Read the model definition and answer for the solid it produces. Units are mm, in the model's axes. Coordinates: 2 decimals unless noted, no trailing zeros. Write each loop counter-clockwise with the first axis right and the second up, starting at its lowest first coordinate (ties: lowest second). Pieces come first, ordered by that corner, then holes. Notation, with made-up numbers: (-24, 35.25) -> (11, 35.25) arc R33 ccw to (11, 69.25) -> close; hole circle Ø8 at (8, 38). An arc over 180 degrees is marked (long way). One line per item, written item: value. Start each with the question number.
1. Given P1, Ø1.5, axis at x = 11, z = 1.5, coming from the +Y side, flat-ended and moving along its own axis, determine where the tip first touches the part or whether it passes through.
2. Find section A-A, the plane x = 6.5. Write down the section's boundary in (y, z).
3. Consider line 1 along Y through (x, z) = (1, -0.8); line 2 along Y through (x, z) = (5, -0.1); line 3 along Z through (x, y) = (15, -1.5). Determine where each line is inside the solid, lowest interval first.
Autodesk Inventor part; units mm, degrees
ref_plane "YZ Plane" through (0, 0, 0) normal (1, 0, 0) x (0, 1, 0)
ref_plane "XZ Plane" through (0, 0, 0) normal (0, 1, 0) x (-1, 0, 0)
ref_plane "XY Plane" through (0, 0, 0) normal (0, 0, 1) x (1, 0, 0)
sketch "Skizze" plane through (0, 0, 0) normal (1, 0, 0) x (0, 1, 0)
  circle A0 centre (0, 0) radius 2
  dimension "d1" = 4
extrude "Körper" add sketch "Skizze" along normal blind 16
chamfer "Fase1" distance 0.63 angle 15 1 edges at (0, -2, 0) measured on face at (10.6667, 1.9935, -0.1609)
chamfer "Skizze2" distance 0.63 angle 15 1 edges at (16, -2, 0) measured on face at (10.8767, 1.9935, -0.1609)
equation "\"d1\" = NND"
equation "\"d2\" = NLG"
equation "\"d8\" = PHH"
equation "\"d9\" = FAWI"
equation "\"d12\" = PHH"
equation "\"d4\" = PHH"
equation "\"d5\" = FAWI"
equation "\"d11\" = PHH"
equation "\"NND\" = 4"
equation "\"NLG\" = 16"
equation "\"PHH\" = 0.63"
equation "\"FAWI\" = 15deg"
equation "\"KAH\" = 0"
properties part number "ISO 2338 - 4 m6 x 16" material "Edelstahl, austenitisch"
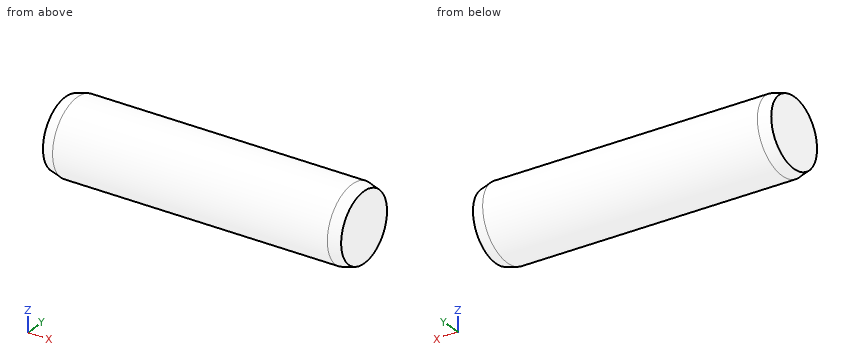
Answer block:
1. P1: stops at y = 1.85
2. outline: circle Ø4 at (0, 0)
3. line 1: y = -1.83 to 1.83
3. line 2: y = -2 to 2
3. line 3: z = -1.32 to 1.32
